Check sheet for the modelled part. Datum: model origin and axes. Units: mm. Give positions to 0.01 mm unless a question says otherwise; leave off trailing zeros. Loops run counter-clockwise (first coordinate to the right, second up) from the corner with the lowest first, then second, coordinate; pieces in that order, holes last. Notation, with made-up numbers: (28.5, 79.25) - (57.5, 79.25) arc R18 ccw to (57.5, 106.25) - close; hole circle Ø4 at (1, 88). An arc over 180 degrees is marked (long way). Use one line per item in the form item = value.
from build123d import *

# Parameters (mm, degrees)
BOSS_EXTRUDE1_DEPTH = 3
SKETCH3_W           = 14
SKETCH3_H           = 3
CUT_EXTRUDE1_DEPTH  = 3
SKETCH7_R           = 20
CUT_EXTRUDE2_DEPTH  = 3
SKETCH9_R           = 1.7
CUT_EXTRUDE3_DEPTH  = 3


with BuildPart() as part:
    # Sketch1 → Boss-Extrude1 (new body)
    with BuildSketch(Plane(origin=(0, 0, 0), x_dir=(0, 0, -1), z_dir=(1, 0, 0))):
        Polygon((-140, 34), (-140, 50), (-124, 50), (-123.5, 42.997828908), (-123, 42.997828908), (-123, 51.997828908), (-123.5, 52.997828908), (-124, 53.497828908), (-124, 54.497828908), (-122.5, 55.997828908), (-121, 55.997828908), (-120.5, 42.997828908), (-120, 42.997828908), (-120, 55.997828908), (-112, 55.997828908), (-112, 42.997828908), (-111.5, 42.997828908), (-111, 55.997828908), (-109.5, 55.997828908), (-108, 54.497828908), (-108, 53.497828908), (-108.5, 52.997828908), (-109, 51.997828908), (-109, 42.997828908), (-108.5, 42.997828908), (-108, 50), (-8, 50), (-7.5, 42.997828908), (-7, 42.997828908), (-7, 51.997828908), (-7.5, 52.997828908), (-8, 53.497828908), (-8, 54.497828908), (-6.5, 55.997828908), (-5, 55.997828908), (-4.5, 42.997828908), (-4, 42.997828908), (-4, 55.997828908), (4, 55.997828908), (4, 42.997828908), (4.5, 42.997828908), (5, 55.997828908), (6.5, 55.997828908), (8, 54.497828908), (8, 53.497828908), (7.5, 52.997828908), (7, 51.997828908), (7, 42.997828908), (7.5, 42.997828908), (8, 50), (108, 50), (108.5, 42.997828908), (109, 42.997828908), (109, 51.997828908), (108.5, 52.997828908), (108, 53.497828908), (108, 54.497828908), (109.5, 55.997828908), (111, 55.997828908), (111.5, 42.997828908), (112, 42.997828908), (112, 55.997828908), (120, 55.997828908), (120, 42.997828908), (120.5, 42.997828908), (121, 55.997828908), (122.5, 55.997828908), (124, 54.497828908), (124, 53.497828908), (123.5, 52.997828908), (123, 51.997828908), (123, 42.997828908), (123.5, 42.997828908), (124, 50), (140, 50), (140, 34), (132.997828908, 33.5), (132.997828908, 33), (141.997828908, 33), (142.997828908, 33.5), (143.497828908, 34), (144.497828908, 34), (145.997828908, 32.5), (145.997828908, 31), (132.997828908, 30.5), (132.997828908, 30), (145.997828908, 30), (145.997828908, 22), (132.997828908, 22), (132.997828908, 21.5), (145.997828908, 21), (145.997828908, 19.5), (144.497828908, 18), (143.497828908, 18), (142.997828908, 18.5), (141.997828908, 19), (132.997828908, 19), (132.997828908, 18.5), (140, 18), (140, -18), (132.997828908, -18.5), (132.997828908, -19), (141.997828908, -19), (142.997828908, -18.5), (143.497828908, -18), (144.497828908, -18), (145.997828908, -19.5), (145.997828908, -21), (132.997828908, -21.5), (132.997828908, -22), (145.997828908, -22), (145.997828908, -30), (132.997828908, -30), (132.997828908, -30.5), (145.997828908, -31), (145.997828908, -32.5), (144.497828908, -34), (143.497828908, -34), (142.997828908, -33.5), (141.997828908, -33), (132.997828908, -33), (132.997828908, -33.5), (140, -34), (140, -56), (-140, -56), (-140, -34), (-132.997828908, -33.5), (-132.997828908, -33), (-141.997828908, -33), (-142.997828908, -33.5), (-143.497828908, -34), (-144.497828908, -34), (-145.997828908, -32.5), (-145.997828908, -31), (-132.997828908, -30.5), (-132.997828908, -30), (-145.997828908, -30), (-145.997828908, -22), (-132.997828908, -22), (-132.997828908, -21.5), (-145.997828908, -21), (-145.997828908, -19.5), (-144.497828908, -18), (-143.497828908, -18), (-142.997828908, -18.5), (-141.997828908, -19), (-132.997828908, -19), (-132.997828908, -18.5), (-140, -18), (-140, 18), (-132.997828908, 18.5), (-132.997828908, 19), (-141.997828908, 19), (-142.997828908, 18.5), (-143.497828908, 18), (-144.497828908, 18), (-145.997828908, 19.5), (-145.997828908, 21), (-132.997828908, 21.5), (-132.997828908, 22), (-145.997828908, 22), (-145.997828908, 30), (-132.997828908, 30), (-132.997828908, 30.5), (-145.997828908, 31), (-145.997828908, 32.5), (-144.497828908, 34), (-143.497828908, 34), (-142.997828908, 33.5), (-141.997828908, 33), (-132.997828908, 33), (-132.997828908, 33.5), align=None)
    extrude(amount=BOSS_EXTRUDE1_DEPTH)

    # Sketch3 → Cut-Extrude1 (cut)
    with BuildSketch(Plane(origin=(3, 0, 0), x_dir=(0, 0, -1), z_dir=(1, 0, 0))):
        with Locations((-116, -51.5)):
            Rectangle(SKETCH3_W, SKETCH3_H)
        with Locations((0, -51.5)):
            Rectangle(SKETCH3_W, SKETCH3_H)
        with Locations((116, -51.5)):
            Rectangle(SKETCH3_W, SKETCH3_H)
    extrude(amount=-CUT_EXTRUDE1_DEPTH, mode=Mode.SUBTRACT)

    # Sketch7 → Cut-Extrude2 (cut)
    with BuildSketch(Plane(origin=(3, 0, 0), x_dir=(0, 0, -1), z_dir=(1, 0, 0))):
        with Locations((-80, 0)):
            Circle(SKETCH7_R)
    extrude(amount=-CUT_EXTRUDE2_DEPTH, mode=Mode.SUBTRACT)

    # Sketch9 → Cut-Extrude3 (cut)
    with BuildSketch(Plane(origin=(3, 0, 0), x_dir=(0, 0, -1), z_dir=(1, 0, 0))):
        with Locations((-96, 16)):
            Circle(SKETCH9_R)
        with Locations((-64, 16)):
            Circle(SKETCH9_R)
        with Locations((-64, -16)):
            Circle(SKETCH9_R)
        with Locations((-96, -16)):
            Circle(SKETCH9_R)
    extrude(amount=-CUT_EXTRUDE3_DEPTH, mode=Mode.SUBTRACT)


solid = part.part
Item 1: Gauge pin test, flat end, axial feed: P1, Ø1.5, axis at x = 2, y = 46.5, coming from the +Z side. Record the tip position at first contact, or that the pin passes through.
Answer block:
P1 = 140
Item 2: Section check C-C on x = 2. Give the number of separate pieces and of enclosed holes in the cut face, then the cut area to 3 significant figures.
Answer block:
separate_pieces = 1
enclosed_holes = 8
area = 28,700 mm2
Item 3: Section check B-B on y = 0. Record the boundary of the cut face in (x, z), then the cut area to 3 significant figures.
Answer block:
outline = (0, -140) - (3, -140) - (3, 60) - (0, 60) - close; (0, 100) - (3, 100) - (3, 140) - (0, 140) - close
area = 720 mm2
Item 4: Section check A-A on z = 80. Record the boundary of the cut face in (x, y), then the cut area to 3 significant figures.
Answer block:
outline = (0, -56) - (3, -56) - (3, -20) - (0, -20) - close; (0, 20) - (3, 20) - (3, 50) - (0, 50) - close
area = 198 mm2
Item 5: Section check D-D on z = -28. Record the boundary of the cut face in (x, y).
Answer block:
outline = (0, -56) - (3, -56) - (3, 50) - (0, 50) - close
Item 6: Thickness scan on L1, parallel to Y at x = 1.1, z = 64; L2, parallel to Y at x = 1.85, z = 80; L3, parallel to Z at x = 0.45, y = 16.5. Record the ranges inside material, lowest first.
Answer block:
L1 = -56 to -17.7, -14.3 to -12, 12 to 14.3, 17.7 to 50
L2 = -56 to -20, 20 to 50
L3 = -140 to 62.38, 65.62 to 68.7, 91.3 to 94.38, 97.62 to 140
Item 7: Mould release check, pull along Z, two halves, no side actions. Record for faces 1 (the face through (1.52, 0.88, 99.98)), 2 (the face through (0, 1, -2)): released by +Z, released by -Z, zero draft, split by the parting line, or undercut.
Answer block:
face_1 = undercut
face_2 = zero draft
